The model under review builds one solid part; all positions refer to its coordinate system, in mm. Face numbers are marked on the shaded views. Give positions to 0.01 mm unless a question says otherwise; leave off trailing zeros. Order: outer loops, then holes, each group sorted by start corner. A loop starts at its lowest first (then second) coordinate and runs counter-clockwise, first axis right, second up. Notation, with made-up numbers: (63, 10.5) - (86, 10.5) arc R19 cw to (86, 26.5) - close; hole circle Ø5 at (-13.75, 67.25). An arc over 180 degrees is marked (long way). Use CSV: the item, a comma, the result in double quotes. Start each with the question number.
```python
from build123d import *

# Parameters (mm, degrees)
SKETCH1_R            = 5
BOSS_EXTRUDE1_DEPTH  = 2
FILLET1_R            = 20
M3_CLEARANCE_HOLE2_D = 3.4
SKETCH5_R            = 0.9
BOSS_EXTRUDE2_DEPTH  = 5
CHAMFER1_SIZE        = 3


with BuildPart() as part:
    # Sketch1 → Boss-Extrude1 (new body)
    with BuildSketch(Plane(origin=(0, 0, 0), x_dir=(1, 0, 0), z_dir=(0, 1, 0))):
        with Locations((21.6, 9)):
            Circle(SKETCH1_R)
        with BuildLine():
            Line((24.81621403, 11.274080729), (33.146482921, 21.191067504))
            ThreePointArc((33.146482921, 21.191067504), (36.129576259, 26.297114594), (31.615073192, 22.477451677))
            Line((31.615073192, 22.477451677), (21.6, 10.554745497))
            Line((21.6, 10.554745497), (11.584926808, 22.477451677))
            ThreePointArc((11.584926808, 22.477451677), (7.070423741, 26.297114594), (10.053517079, 21.191067504))
            Line((10.053517079, 21.191067504), (18.38378597, 11.274080729))
            Line((18.38378597, 11.274080729), (5.257510753, 16.196433936))
            ThreePointArc((5.257510753, 16.196433936), (-2.46531671, 18.024493766), (4.55526387, 14.323775581))
            Line((4.55526387, 14.323775581), (18.751998752, 9))
            Line((18.751998752, 9), (4.55526387, 3.676224419))
            ThreePointArc((4.55526387, 3.676224419), (-2.46531671, -0.024493766), (5.257510753, 1.803566064))
            Line((5.257510753, 1.803566064), (18.38378597, 6.725919271))
            Line((18.38378597, 6.725919271), (10.053517079, -3.191067504))
            ThreePointArc((10.053517079, -3.191067504), (7.070423741, -8.297114594), (11.584926808, -4.477451677))
            Line((11.584926808, -4.477451677), (21.6, 7.445254503))
            Line((21.6, 7.445254503), (31.615073192, -4.477451677))
            ThreePointArc((31.615073192, -4.477451677), (36.129576259, -8.297114594), (33.146482921, -3.191067504))
            Line((33.146482921, -3.191067504), (24.81621403, 6.725919271))
            Line((24.81621403, 6.725919271), (37.942489247, 1.803566064))
            ThreePointArc((37.942489247, 1.803566064), (45.66531671, -0.024493766), (38.64473613, 3.676224419))
            Line((38.64473613, 3.676224419), (24.448001248, 9))
            Line((24.448001248, 9), (38.64473613, 14.323775581))
            ThreePointArc((38.64473613, 14.323775581), (45.66531671, 18.024493766), (37.942489247, 16.196433936))
            Line((37.942489247, 16.196433936), (24.81621403, 11.274080729))
        make_face()
    extrude(amount=BOSS_EXTRUDE1_DEPTH)

    # Fillet1
    fillet1_edges = [part.edges().sort_by_distance(p)[0] for p in [
        (5.257510753, 1, -16.196433936),
        (4.55526387, 1, -14.323775581),
        (4.55526387, 1, -3.676224419),
        (5.257510753, 1, -1.803566064),
        (10.053517079, 1, 3.191067504),
        (11.584926808, 1, 4.477451677),
        (31.615073192, 1, 4.477451677),
        (33.146482921, 1, 3.191067504),
        (37.942489247, 1, -1.803566064),
        (38.64473613, 1, -3.676224419),
        (38.64473613, 1, -14.323775581),
        (37.942489247, 1, -16.196433936),
        (33.146482921, 1, -21.191067504),
        (31.615073192, 1, -22.477451677),
        (11.584926808, 1, -22.477451677),
        (10.053517079, 1, -21.191067504),
    ]]
    fillet(fillet1_edges, radius=FILLET1_R)

    # M3 Clearance Hole2 (through all)
    with Locations(Plane(origin=(0, 2, 0), x_dir=(1, 0, 0), z_dir=(0, 1, 0))):
        with Locations((9, -6), (34.2, -6), (34.2, 24), (9, 24)):
            Hole(M3_CLEARANCE_HOLE2_D / 2)

    # Sketch5 → Boss-Extrude2 (add)
    with BuildSketch(Plane(origin=(0, 2, 0), x_dir=(1, 0, 0), z_dir=(0, 1, 0))):
        with Locations(Location((1.28, 1.38, 0), (0, 0, 270))):
            Circle(SKETCH5_R)
        with Locations(Location((41.92, 1.38, 0), (0, 0, 270))):
            Circle(SKETCH5_R)
        with Locations(Location((41.92, 16.62, 0), (0, 0, 270))):
            Circle(SKETCH5_R)
        with Locations(Location((1.28, 16.62, 0), (0, 0, 270))):
            Circle(SKETCH5_R)
    extrude(amount=BOSS_EXTRUDE2_DEPTH)

    # Chamfer1
    chamfer1_edges = [part.edges().sort_by_distance(p)[0] for p in [
        (1.28, 2, -2.28),
        (41.92, 2, -2.28),
        (41.92, 2, -17.52),
        (1.28, 2, -17.52),
    ]]
    chamfer(chamfer1_edges, length=CHAMFER1_SIZE)


solid = part.part
```
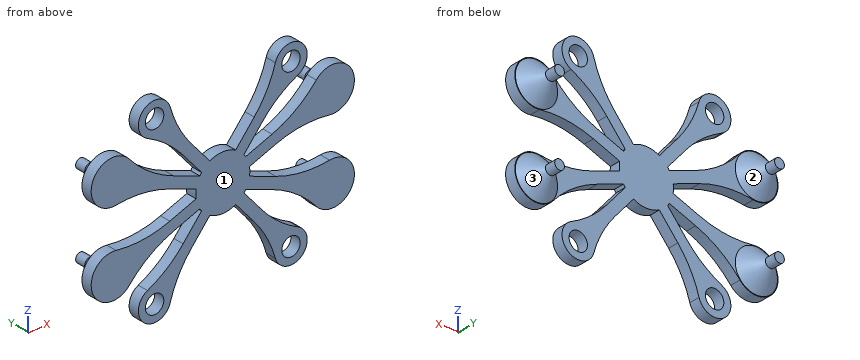
1. To check wall thickness, follow L1, parallel to Z at x = 9, y = 0.7; L2, parallel to X at y = 1.3, z = 6; L3, parallel to Z at x = 17, y = 0.5. State the ranges of each line that lie inside material, in increasing order. Write a range as [from, to].
2. Consider section B-B (x = 33.5). Give the boundary of the cut face in (y, z), and give its area (3 significant figures).
3. Mouldability with a two-part tool opening along Z and no side actions: class the marked faces 1, 2 and 3 as pulls with the +Z half, pulls with the -Z half, needs draft (parallel to the pull), parting line crosses it, or undercut.
4. Clearance check with flat-ended pins moving along their axes: pin 1 (5.5 mm diameter, centred on x = 9, z = -24, fed in from +Y); pin 2 (2 mm diameter, centred on y = 2, z = -5, fed in from +X); pin 3 (2 mm diameter, centred on x = 28, y = 2, fed in from +Z). State where each tip first meets the part, or that it passes through.
5. Consider section D-D (z = -24). Give the boundary of the cut face in (x, y).
6. Consider section C-C (y = 6). Give the boundary of the cut face in (x, z).
7. Consider section A-A (x = 41.92). Give the boundary of the cut face in (y, z), and give its area (3 significant figures).
Answers follow:
1,L1,"z = [-27, -25.7], [-22.3, -20.6], [-15.2, -12.43], [-5.57, -2.8], [2.6, 4.3], [7.7, 9]"
1,L2,"x = [6, 7.3], [10.7, 12.14], [31.06, 32.5], [35.9, 37.2]"
1,L3,"z = [-16.03, -12.92], [-11.79, -6.21], [-5.08, -1.97]"
2,outline,"(0, -26.92) - (2, -26.92) - (2, -25.55) - (0, -25.55) - close; (0, -22.45) - (2, -22.45) - (2, -20.18) - (0, -20.18) - close; (0, -14.79) - (2, -14.79) - (2, -12.26) - (0, -12.26) - close; (0, -5.74) - (2, -5.74) - (2, -3.21) - (0, -3.21) - close; (0, 2.18) - (2, 2.18) - (2, 4.45) - (0, 4.45) - close; (0, 7.55) - (2, 7.55) - (2, 8.92) - (0, 8.92) - close"
2,area,"24.7 mm^2"
3,face 1,"needs draft"
3,face 2,"undercut"
3,face 3,"undercut"
4,pin 1,"stops at y = 2"
4,pin 2,"stops at x = 44.94"
4,pin 3,"stops at z = 1.65"
5,outline,"(6, 0) - (7.3, 0) - (7.3, 2) - (6, 2) - close; (10.7, 0) - (12.14, 0) - (12.14, 2) - (10.7, 2) - close; (31.06, 0) - (32.5, 0) - (32.5, 2) - (31.06, 2) - close; (35.9, 0) - (37.2, 0) - (37.2, 2) - (35.9, 2) - close"
6,outline,"circle Ø1.8 at (1.28, -16.62); circle Ø1.8 at (1.28, -1.38); circle Ø1.8 at (41.92, -16.62); circle Ø1.8 at (41.92, -1.38)"
7,outline,"(0, -20.62) - (2, -20.62) - (2, -20.52) - (5, -17.52) - (7, -17.52) - (7, -15.72) - (5, -15.72) - (2, -12.72) - (2, -12.62) - (0, -12.62) - close; (0, -5.38) - (2, -5.38) - (2, -5.28) - (5, -2.28) - (7, -2.28) - (7, -0.48) - (5, -0.48) - (2, 2.52) - (2, 2.62) - (0, 2.62) - close"
7,area,"68.0 mm^2"
